from build123d import *

# Parameters (mm, degrees)
SKETCH1_R           = 1.6
BOSS_EXTRUDE1_DEPTH = 15


with BuildPart() as part:
    # Sketch1 → Boss-Extrude1 (new body)
    with BuildSketch(Plane(origin=(0, 0, 0), x_dir=(1, 0, 0), z_dir=(0, 1, 0))):
        with BuildLine():
            Line((-16, -18), (16, -18))
            ThreePointArc((16, -18), (18.828427125, -16.828427125), (20, -14))
            Line((20, -14), (20, 14))
            ThreePointArc((20, 14), (18.828427125, 16.828427125), (16, 18))
            Line((16, 18), (-16, 18))
            ThreePointArc((-16, 18), (-18.828427125, 16.828427125), (-20, 14))
            Line((-20, 14), (-20, -14))
            ThreePointArc((-20, -14), (-18.828427125, -16.828427125), (-16, -18))
        make_face()
        with Locations((16, 14)):
            Circle(SKETCH1_R, mode=Mode.SUBTRACT)
        with Locations((-16, 14)):
            Circle(SKETCH1_R, mode=Mode.SUBTRACT)
        with Locations((-16, -14)):
            Circle(SKETCH1_R, mode=Mode.SUBTRACT)
        with Locations((16, -14)):
            Circle(SKETCH1_R, mode=Mode.SUBTRACT)
    extrude(amount=BOSS_EXTRUDE1_DEPTH)


solid = part.part
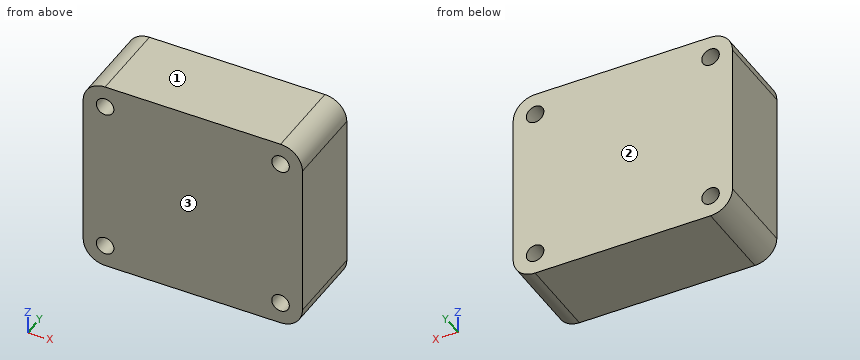
For this review, take the finished solid that the model builds, in its own axes (mm). Face numbers are marked on the shaded views. Round coordinates to 2 decimals unless told otherwise and drop trailing zeros. Loops run counter-clockwise (first coordinate to the right, second up) from the corner with the lowest first, then second, coordinate; pieces in that order, holes last. Notation, with made-up numbers: (50.5, 42.5) - (87.5, 42.5) arc R21 cw to (87.5, 56.5) - close; hole circle Ø8 at (84.5, -13). An arc over 180 degrees is marked (long way). Put each result on its own line as item: value. Start each with the question number.
1. For probe 1 along Z at (x, y) = (16, 10.75); probe 2 along X at (y, z) = (4.25, 14); probe 3 along X at (y, z) = (13.25, -15), list the stretches that pass through material, from the lowest coordinate up. Write a range as [from, to].
2. Consider section A-A on y = 9.5. State the section outline as (x, z) points.
3. Mouldability with a two-part tool opening along Y and no side actions: class the marked faces 1, 2 and 3 as +Y half, -Y half, draft (parallel to the pull), parting line (faces both ways), or undercut.
Result sheet:
1. probe 1: [-18, -15.6], [-12.4, 12.4], [15.6, 18]
1. probe 2: [-20, -17.6], [-14.4, 14.4], [17.6, 20]
1. probe 3: [-19.87, -17.25], [-14.75, 14.75], [17.25, 19.87]
2. outline: (-20, -14) arc R4 ccw to (-16, -18) - (16, -18) arc R4 ccw to (20, -14) - (20, 14) arc R4 ccw to (16, 18) - (-16, 18) arc R4 ccw to (-20, 14) - close; hole circle Ø3.2 at (-16, -14); hole circle Ø3.2 at (-16, 14); hole circle Ø3.2 at (16, -14); hole circle Ø3.2 at (16, 14)
3. face 1: draft
3. face 2: +Y half
3. face 3: -Y half
